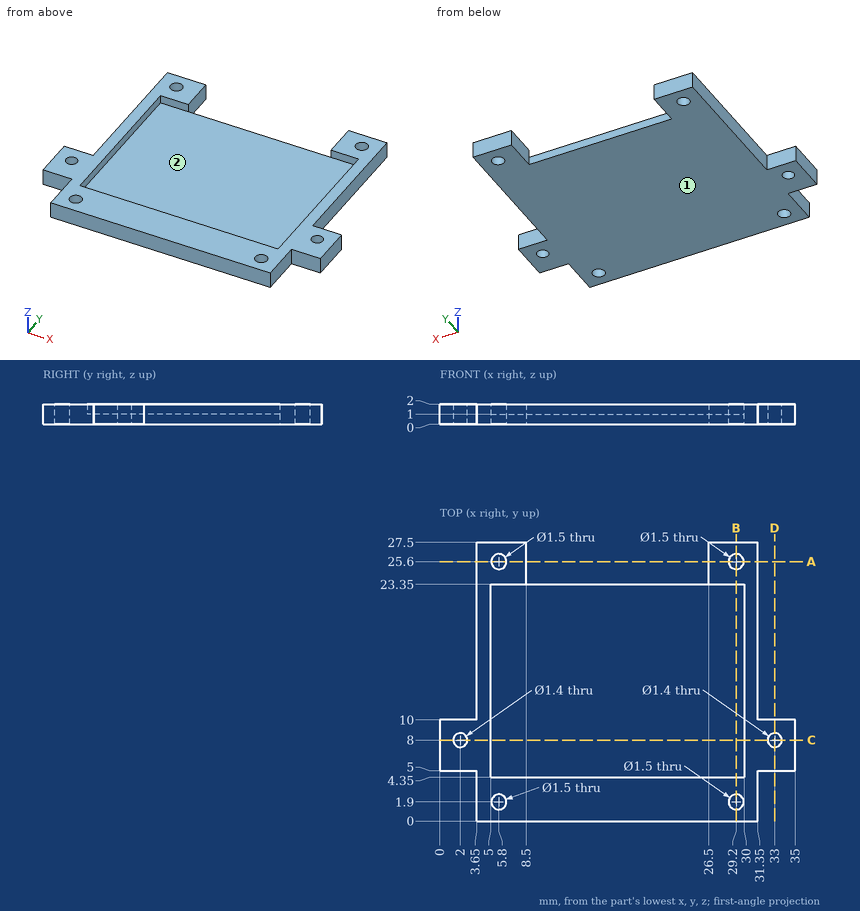
Source: three-view drawing plus pictorial views. Frame: mm from the lowest corner of the part. Give positions to 0.01 mm unless a question says otherwise; leave off trailing zeros. Loops run counter-clockwise (first coordinate to the right, second up) from the corner with the lowest first, then second, coordinate; pieces in that order, holes last. Notation, with made-up numbers: (52.5, 60) -> (102.5, 60) arc R19 ccw to (102.5, 86) -> close; hole circle Ø1 at (1.5, -3). An arc over 180 degrees is marked (long way). Put each result on its own line as item: value. Start each with the question number.
1) Contact query for flat-ended pins moving along their axis: P1, Ø0.5, axis at x = 19.5, z = 0.5, coming from the +Y side; P2, Ø0.6, axis at y = 2, z = 1, coming from the -X side. Output: stop coordinate, or through.
2) Cut plane C-C (y = 8). Return loops of the section in (x, z), then the cut area to 3 significant figures.
3) Material intervals for probe 1 along Y at (x, z) = (29.2, 1.3); probe 2 along X at (y, z) = (25.6, 1.15); probe 3 along X at (y, z) = (17, 1.55), sorted ascending.
4) Cut plane D-D (x = 33). Return loops of the section in (y, z).
5) Draft query along X for the marked faces 1 and 2. Return one class per face: released by +X, released by -X, zero draft, split by the parting line, or undercut.
6) Cut plane B-B (x = 29.2). Return loops of the section in (y, z).
7) Cut plane A-A (y = 25.6). Return loops of the section in (x, z), then the cut area to 3 significant figures.
Results are:
1. P1: stops at y = 23.35
1. P2: stops at x = 3.65
2. outline: (0, 0) -> (1.3, 0) -> (1.3, 2) -> (0, 2) -> close; (2.7, 0) -> (32.3, 0) -> (32.3, 2) -> (30, 2) -> (30, 1) -> (5, 1) -> (5, 2) -> (2.7, 2) -> close; (33.7, 0) -> (35, 0) -> (35, 2) -> (33.7, 2) -> close
2. area: 39.4 mm2
3. probe 1: y = 0 to 1.15, 2.65 to 4.35, 23.35 to 24.85, 26.35 to 27.5
3. probe 2: x = 3.65 to 5.05, 6.55 to 8.5, 26.5 to 28.45, 29.95 to 31.35
3. probe 3: x = 3.65 to 5, 30 to 31.35
4. outline: (5, 0) -> (7.3, 0) -> (7.3, 2) -> (5, 2) -> close; (8.7, 0) -> (10, 0) -> (10, 2) -> (8.7, 2) -> close
5. face 1: zero draft
5. face 2: undercut
6. outline: (0, 0) -> (1.15, 0) -> (1.15, 2) -> (0, 2) -> close; (2.65, 0) -> (24.85, 0) -> (24.85, 2) -> (23.35, 2) -> (23.35, 1) -> (4.35, 1) -> (4.35, 2) -> (2.65, 2) -> close; (26.35, 0) -> (27.5, 0) -> (27.5, 2) -> (26.35, 2) -> close
7. outline: (3.65, 0) -> (5.05, 0) -> (5.05, 2) -> (3.65, 2) -> close; (6.55, 0) -> (8.5, 0) -> (8.5, 2) -> (6.55, 2) -> close; (26.5, 0) -> (28.45, 0) -> (28.45, 2) -> (26.5, 2) -> close; (29.95, 0) -> (31.35, 0) -> (31.35, 2) -> (29.95, 2) -> close
7. area: 13.4 mm2
